Build history of the part. All positions in model axes, mm. A direction names the side the tool comes from. Round coordinates to 2 decimals unless told otherwise and drop trailing zeros. Write each loop counter-clockwise with the first axis right and the second up, starting at its lowest first coordinate (ties: lowest second). Pieces come first, ordered by that corner, then holes. Notation, with made-up numbers: (41.25, -6) - (86.25, -6) arc R25 cw to (86.25, 29) - close; hole circle Ø4 at (20, 54.5). An arc over 180 degrees is marked (long way). One line per question, with ' | ' between items.
from build123d import *

# Parameters (mm, degrees)
SKETCH_R     = 17
PAD_DEPTH    = 35
SKETCH001_R  = 12
PAD001_DEPTH = 150
SKETCH002_R  = 8.5
PAD002_DEPTH = 30
SKETCH003_R  = 6.5
POCKET_DEPTH = 17


with BuildPart() as part:
    # Sketch → Pad (new body)
    with BuildSketch(Plane.XY):
        Circle(SKETCH_R)
    extrude(amount=PAD_DEPTH)

    # Sketch001 (on Face2 of Pad) → Pad001 (join)
    with BuildSketch(Plane(origin=(0, 0, 0), x_dir=(1, 0, 0), z_dir=(0, 0, -1))):
        Circle(SKETCH001_R)
    extrude(amount=PAD001_DEPTH)

    # Sketch002 (on Face5 of Pad001) → Pad002 (join)
    with BuildSketch(Plane(origin=(0, 0, -150), x_dir=(1, 0, 0), z_dir=(0, 0, -1))):
        Circle(SKETCH002_R)
    extrude(amount=PAD002_DEPTH)

    # Sketch003 (on DatumPlane) → Pocket (cut, symmetric)
    with BuildSketch(Plane(origin=(0, 0, 35), x_dir=(1, 0, 0), z_dir=(0, -1, 0))):
        with Locations((0, -17.5)):
            Circle(SKETCH003_R)
    extrude(amount=POCKET_DEPTH, both=True, mode=Mode.SUBTRACT)


solid = part.part
Q1. Saw through at C-C, the plane z = -39.5. List the corners of the cut face in (x, y), then the cut area to 3 significant figures.
Found:
outline: circle Ø24 at (0, 0) | area: 452 mm^2
Q2. Saw through at B-B, the plane x = 0. List the corners of the cut face in (y, z), then the cut area to 3 significant figures.
Found:
outline: (-17, 0) - (-12, 0) - (-12, -150) - (-8.5, -150) - (-8.5, -180) - (8.5, -180) - (8.5, -150) - (12, -150) - (12, 0) - (17, 0) - (17, 11) - (-17, 11) - close; (-17, 24) - (17, 24) - (17, 35) - (-17, 35) - close | area: 4,860 mm^2
Q3. Pull direction Z, two halves, no side cores. Call faces 1 (the flat face through (0, 0, 35)), 2 (the flat face through (-8.2, -2.8, -150)), 3 (the cylindrical face through (-0.846, -0.238, 23.945)), 4 (the cylindrical face through (-11.99, -0.53, -73.95)): +Z half, -Z half, draft (parallel to the pull), parting line (faces both ways), or undercut.
Found:
face 1: +Z half | face 2: -Z half | face 3: undercut | face 4: draft
Q4. Saw through at D-D, the plane z = 17.5. List the corners of the cut face in (x, y).
Found:
outline: (-6.5, -15.71) - (-6.5, 15.71) arc R17 ccw to start; (6.5, -15.71) arc R17 ccw to (6.5, 15.71) - close
Q5. Saw through at A-A, the plane y = 0. List the corners of the cut face in (x, z).
Found:
outline: (-17, 0) - (-12, 0) - (-12, -150) - (-8.5, -150) - (-8.5, -180) - (8.5, -180) - (8.5, -150) - (12, -150) - (12, 0) - (17, 0) - (17, 35) - (-17, 35) - close; hole circle Ø13 at (0, 17.5)
Q6. Which spindle directions (+Z, -Z, +X, -X, +Y, -Y) get a long thin tool onto all of the face, cutting with end or side? Do faces 5 (the cylindrical face through (4.57, -7.167, -164.79)), 6 (the cylindrical face through (16.215, 5.106, 17.255)). Say none if no direction does.
Found:
face 5: -Z | face 6: +Z, -Z
Q7. Drop flat-ended pins along their axis: pin 1 (5 mm diameter, centred on y = 0.5, z = -80.5, fed in from +X); pin 2 (10 mm diameter, centred on y = -10.5, z = -67, fed in from -X); pin 3 (5 mm diameter, centred on x = 6, z = 6, fed in from +Y); pin 4 (8 mm diameter, centred on x = 0, z = 17.5, fed in from +Y) (3 decimals). Give the stop position or say it passes through.
Found:
pin 1: x = 12 | pin 2: x = -10.67 | pin 3: y = 16.64 | pin 4: through
Q8. Drill centre lines: L1, parallel to Z at x = 0, y = 6; L2, parallel to Y at x = -0.5, z = -58; L3, parallel to Z at x = 13.5, y = 1.5. Where is each one in solid material? Low to high. Write a range as from..to.
Found:
L1: -180..11, 24..35 | L2: -11.99..11.99 | L3: 0..35
